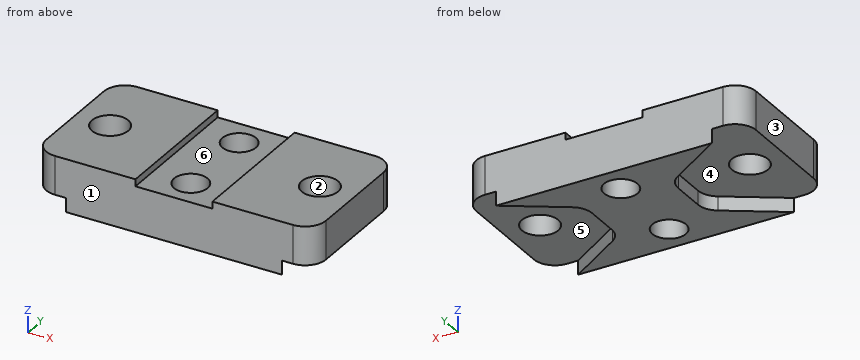
from build123d import *

# Parameters (mm, degrees)
SKETCH_W        = 40
SKETCH_H        = 20
SKETCH_R        = 2.6
PAD_DEPTH       = 7.5
POCKET001_DEPTH = 2
SKETCH003_W     = 11
SKETCH003_H     = 1
POCKET_DEPTH    = 20.001
SKETCH004_R     = 2.4
POCKET002_DEPTH = 7.501
FILLET_R        = 3


with BuildPart() as part:
    # Sketch → Pad (new body)
    with BuildSketch(Plane.XY):
        Rectangle(SKETCH_W, SKETCH_H)
        with Locations((-15, 0)):
            Circle(SKETCH_R, mode=Mode.SUBTRACT)
        with Locations((15, 0)):
            Circle(SKETCH_R, mode=Mode.SUBTRACT)
    extrude(amount=PAD_DEPTH)

    # Sketch002 → Pocket001 (cut)
    with BuildSketch(Plane(origin=(0, 0, 0), x_dir=(1, 0, 0), z_dir=(0, 0, -1))):
        Polygon((20.661249, -13.364706), (20.661249, 13.364706), (6.159635, 4.022958), (6.159635, -4.022958), align=None)
    pocket001 = extrude(amount=-POCKET001_DEPTH, mode=Mode.SUBTRACT)

    # Mirrored: Pocket001 across Sketch002 V_Axis
    add(pocket001.mirror(Plane(origin=(0, 0, 0), x_dir=(0, 0, -1), z_dir=(1, 0, 0))), mode=Mode.SUBTRACT)

    # Sketch003 (on DatumPlane) → Pocket (cut, through all)
    with BuildSketch(Plane(origin=(0, 10, 0), x_dir=(-1, 0, 0), z_dir=(0, 1, 0))):
        with Locations((0, 7)):
            Rectangle(SKETCH003_W, SKETCH003_H)
    extrude(amount=-POCKET_DEPTH, mode=Mode.SUBTRACT)

    # Sketch004 (on DatumPlane) → Pocket002 (cut, through all)
    with BuildSketch(Plane(origin=(0, 0, 0), x_dir=(1, 0, 0), z_dir=(0, 0, -1))):
        with Locations((0, 5.879738)):
            Circle(SKETCH004_R)
        with Locations((0, -5.879738)):
            Circle(SKETCH004_R)
    extrude(amount=-POCKET002_DEPTH, mode=Mode.SUBTRACT)

    # Fillet
    fillet_edges = [part.edges().sort_by_distance(p)[0] for p in [
        (-6.159635, -4.022958, 1),
        (-6.159635, 4.022958, 1),
        (6.159635, -4.022958, 1),
        (6.159635, 4.022958, 1),
        (20, 10, 4.75),
        (20, -10, 4.75),
        (-20, 10, 4.75),
        (-20, -10, 4.75),
    ]]
    fillet(fillet_edges, radius=FILLET_R)


solid = part.part
The model under review builds one solid part; all positions refer to its coordinate system, in mm. Face numbers are marked on the shaded views. A direction names the side the tool comes from. Round coordinates to 2 decimals unless told otherwise and drop trailing zeros. Loops run counter-clockwise (first coordinate to the right, second up) from the corner with the lowest first, then second, coordinate; pieces in that order, holes last. Notation, with made-up numbers: (16, -6) -> (41, -6) arc R3 cw to (41, -2) -> close; hole circle Ø1 at (89, 8). An arc over 180 degrees is marked (long way). Return JSON: item names as keys, results as strings.
(1) For the marked faces 4, 5 and 6, list the 3-axis set-ups (+Z, -Z, +X, -X, +Y, -Y) from which the entire face can be reached by the end or side of a thin tool; tool diameter is ignored.
Solved:
{"face 4": "-Z, -X", "face 5": "-Z, +X", "face 6": "+Z, +Y, -Y"}
(2) For pin 1 (7 mm diameter, centred on x = -15, y = 0, fed in from -Z); pin 2 (2 mm diameter, centred on y = 0, z = 0.5, fed in from -X); pin 3 (4 mm diameter, centred on x = 15, y = 0, fed in from -Z); pin 4 (1.6 mm diameter, centred on y = -1, z = 1, fed in from +X), all flat-tipped, find the tip position at first contact; note any pin that passes through.
Solved:
{"pin 1": "z = 2", "pin 2": "x = -6.16", "pin 3": "through", "pin 4": "x = 6.16"}
(3) Add section D-D on z = 1.5. Write out the cut boundary in (x, y) (3 decimals).
Solved:
{"outline": "(-15.438, -10) -> (15.438, -10) -> (7.535, -4.909) arc R3 cw to (6.16, -2.387) -> (6.16, 2.387) arc R3 cw to (7.535, 4.909) -> (15.438, 10) -> (-15.438, 10) -> (-7.535, 4.909) arc R3 cw to (-6.16, 2.387) -> (-6.16, -2.387) arc R3 cw to (-7.535, -4.909) -> close; hole circle Ø4.8 at (0, -5.88); hole circle Ø4.8 at (0, 5.88)"}
(4) For line 1 (X direction, y = 0, z = 5.4); line 2 (Y direction, x = 0, z = 3); line 3 (X direction, y = -1.75, z = 5.5), list the stretches that pass through material, from the lowest coordinate up.
Solved:
{"line 1": "-20 to -17.6, -12.4 to 12.4, 17.6 to 20", "line 2": "-10 to -8.28, -3.48 to 3.48, 8.28 to 10", "line 3": "-20 to -16.92, -13.08 to 13.08, 16.92 to 20"}
(5) Add section B-B on y = 0. Write out the cut boundary in (x, z).
Solved:
{"outline": "(-20, 2) -> (-17.6, 2) -> (-17.6, 7.5) -> (-20, 7.5) -> close; (-12.4, 2) -> (-6.16, 2) -> (-6.16, 0) -> (6.16, 0) -> (6.16, 2) -> (12.4, 2) -> (12.4, 7.5) -> (5.5, 7.5) -> (5.5, 6.5) -> (-5.5, 6.5) -> (-5.5, 7.5) -> (-12.4, 7.5) -> close; (17.6, 2) -> (20, 2) -> (20, 7.5) -> (17.6, 7.5) -> close"}
(6) The part is to be moulded in two halves that separate along X. For the marked faces 1, 2 and 3, say which applies: released by +X, released by -X, zero draft, split by the parting line, or undercut.
Solved:
{"face 1": "zero draft", "face 2": "undercut", "face 3": "released by -X"}
(7) Add section A-A on x = 0. Write out the cut boundary in (y, z).
Solved:
{"outline": "(-10, 0) -> (-8.28, 0) -> (-8.28, 6.5) -> (-10, 6.5) -> close; (-3.48, 0) -> (3.48, 0) -> (3.48, 6.5) -> (-3.48, 6.5) -> close; (8.28, 0) -> (10, 0) -> (10, 6.5) -> (8.28, 6.5) -> close"}
(8) Add section C-C on y = -5.5. Write out the cut boundary in (x, z), plus the area to 3 significant figures.
Solved:
{"outline": "(-20, 2) -> (-8.45, 2) -> (-8.45, 0) -> (-2.37, 0) -> (-2.37, 6.5) -> (-5.5, 6.5) -> (-5.5, 7.5) -> (-20, 7.5) -> close; (2.37, 0) -> (8.45, 0) -> (8.45, 2) -> (20, 2) -> (20, 7.5) -> (5.5, 7.5) -> (5.5, 6.5) -> (2.37, 6.5) -> close", "area": "212 mm2"}
